Read the model definition and answer for the solid it produces. Units are mm, in the model's axes. A direction names the side the tool comes from. Coordinates: 2 decimals unless noted, no trailing zeros. Loops run counter-clockwise (first coordinate to the right, second up) from the corner with the lowest first, then second, coordinate; pieces in that order, holes last. Notation, with made-up numbers: (-16.75, -37) -> (19.25, -37) arc R18 ccw to (19.25, -14) -> close; hole circle Ø3 at (68, 29.5). An arc over 180 degrees is marked (long way). One line per question, with ' | ' between items. Start each with the question number.
Autodesk Inventor part; units mm, degrees
ref_plane "YZ Plane" through (0, 0, 0) normal (1, 0, 0) x (0, 1, 0)
ref_plane "XZ Plane" through (0, 0, 0) normal (0, 1, 0) x (-1, 0, 0)
ref_plane "XY Plane" through (0, 0, 0) normal (0, 0, 1) x (1, 0, 0)
sketch "Sketch1" plane through (0, 0, 0) normal (0, 1, 0) x (-1, 0, 0)
  line L0 (-13.3, 9.8) -> (13.3, 9.8)
  line L1 (13.3, 9.8) -> (13.3, -9.8)
  line L2 (13.3, -9.8) -> (-13.3, -9.8)
  line L3 (-13.3, -9.8) -> (-13.3, 9.8)
  line L4 (-13.3, 9.8) -> (13.3, -9.8) construction
  line L5 (13.3, 9.8) -> (-13.3, -9.8) construction
  point P0 (0, 0)
  dimension "d0" = 26.6
  dimension "d1" = 19.6
extrude "Extrusion1" add sketch "Sketch1" along normal blind 1
sketch "Sketch2" plane through (0, 0, 0) normal (0, -1, 0) x (1, 0, 0)
  line L0 (13.3, 9.8) -> (-13.3, 9.8)
  line L1 (13.3, -9.8) -> (13.3, 9.8)
  line L2 (-14.3, -10.8) -> (14.3, -10.8)
  line L3 (14.3, -10.8) -> (14.3, 10.8)
  line L4 (14.3, 10.8) -> (-14.3, 10.8)
  line L5 (-14.3, 10.8) -> (-14.3, -10.8)
  line L6 (-14.3, -10.8) -> (14.3, 10.8) construction
  line L7 (14.3, -10.8) -> (-14.3, 10.8) construction
  point P0 (0, 0)
  dimension "d4" = 1
  dimension "d5" = 1
extrude "Extrusion2" add sketch "Sketch2" along normal blind 1
chamfer "Chamfer1" distance 1 angle 45 4 edges at (0, 0, 10.8) (-14.3, 0, 0) (14.3, 0, 0) (0, 0, -10.8)
properties part number "wysw trans"
(1) Each of these flat-tipped pins is pushed along its axis until it touches: pin 1 Ø0.8 at (y, z) = (0.5, -1.5) entering from +X; pin 2 Ø0.8 at (x, y) = (-5, 0.5) entering from -Z; pin 3 Ø1.1 at (x, y) = (-0.5, 0.5) entering from +Z. Where does it stop, or does it pass through?
(2) A tool of negligible diameter and unlimited length cuts with its end or side. For faces 1 (the flat face through (-0.2, 0.5, -9.8)), 2 (the flat face through (0.2, 0.5, 9.8)), 3 (the flat face through (0, 1, 0)), 4 (the flat face through (13.3, 0.5, -0.1)), 5 (the flat face through (-13.3, 0.5, 0.1)), from which of +Z, -Z, +X, -X, +Y, -Y can it reach the whole face along a straight path? Write none if from no direction.
(3) Section C-C on y = -0.55 is taken. Write down the section's boundary in (x, z).
(4) Find the intervals of material crossed by probe 1 along Z at (x, y) = (4.25, 0); probe 2 along X at (y, z) = (0.25, -7); probe 3 along Z at (x, y) = (5.75, -0.4), in increasing order. Write a range as from..to.
Working result:
1) pin 1: stops at x = 13.3 | pin 2: stops at z = -9.8 | pin 3: stops at z = 9.85
2) face 1: -Z, +X, -X, +Y | face 2: +Z, +X, -X, +Y | face 3: +Z, -Z, +X, -X, +Y | face 4: +Z, -Z, +X, +Y | face 5: +Z, -Z, -X, +Y
3) outline: (-13.85, -10.35) -> (13.85, -10.35) -> (13.85, 10.35) -> (-13.85, 10.35) -> close
4) probe 1: z = -9.8..9.8 | probe 2: x = -13.3..13.3 | probe 3: z = -10.2..10.2
